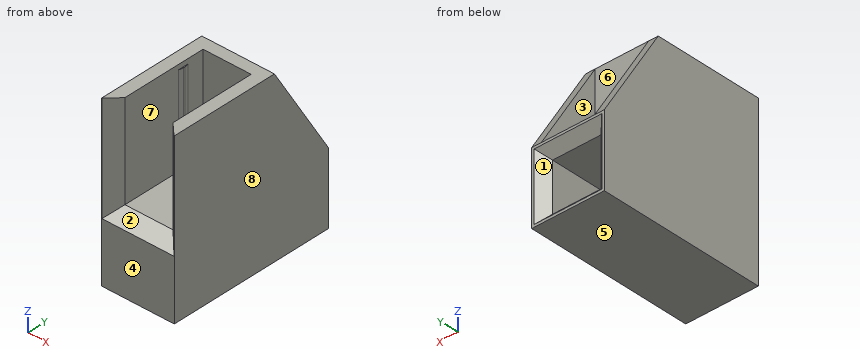
```python
from build123d import *

# Parameters (mm, degrees)
CROQUIS2_W               = 30.3
CROQUIS2_H               = 70
SALIENTE_EXTRUIR2_DEPTH  = 5
SALIENTE_EXTRUIR3_START  = -20
SALIENTE_EXTRUIR3_DEPTH  = 70
SALIENTE_EXTRUIR4_START  = -20
CROQUIS4_W               = 20.2
CROQUIS4_H               = 20.2
SALIENTE_EXTRUIR4_DEPTH  = 4
CHAFL_N4_SIZE            = 4
CROQUIS6_W               = 30.3
CROQUIS6_H               = 5
CROQUIS6_W_2             = 5.125
CROQUIS6_H_2             = 40.5
SALIENTE_EXTRUIR6_DEPTH  = 40
SALIENTE_EXTRUIR7_START  = -15.15
SALIENTE_EXTRUIR7_DEPTH  = 30.3
CROQUIS8_W               = 22.3
CROQUIS8_H               = 24.5
CORTAR_EXTRUIR1_DEPTH    = 40
CHAFL_N9_SIZE            = 5
SALIENTE_EXTRUIR9_DEPTH  = 0.4
REDONDEO3_R              = 5
SALIENTE_EXTRUIR10_DEPTH = 0.4
REDONDEO4_R              = 5


with BuildPart() as part:
    # Croquis2 → Saliente-Extruir2 (new body)
    with BuildSketch(Plane.XY):
        with Locations((0, 15)):
            Rectangle(CROQUIS2_W, CROQUIS2_H)
    extrude(amount=-SALIENTE_EXTRUIR2_DEPTH)

    # Croquis3 → Saliente-Extruir3 (add)
    with BuildSketch(Plane(origin=(0, 0, 0), x_dir=(1, 0, 0), z_dir=(0, 1, 0)).offset(SALIENTE_EXTRUIR3_START)):
        Polygon((-15.15, 30.25), (-15.15, 5), (-10.1, 5), (-10.1, 25.2), (10.1, 25.2), (10.1, 5), (15.15, 5), (15.15, 30.25), align=None)
    extrude(amount=SALIENTE_EXTRUIR3_DEPTH)

    # Croquis4 → Saliente-Extruir4 (add)
    with BuildSketch(Plane(origin=(0, 0, 0), x_dir=(1, 0, 0), z_dir=(0, 1, 0)).offset(SALIENTE_EXTRUIR4_START)):
        with Locations((0, 15.1)):
            Rectangle(CROQUIS4_W, CROQUIS4_H)
    extrude(amount=SALIENTE_EXTRUIR4_DEPTH)

    # Chaflán4
    chafl_n4_edges = [part.edges().sort_by_distance(p)[0] for p in [
        (0, 50, -5),
        (10.1, 50, -15.1),
        (0, 50, -25.2),
        (-10.1, 50, -15.1),
    ]]
    chamfer(chafl_n4_edges, length=CHAFL_N4_SIZE)

    # Croquis6 → Saliente-Extruir6 (add)
    with BuildSketch(Plane.XY):
        with Locations((0, 23)):
            Rectangle(CROQUIS6_W, CROQUIS6_H)
        with Locations((-12.5875, 0.25)):
            Rectangle(CROQUIS6_W_2, CROQUIS6_H_2)
        with Locations((12.5875, 0.25)):
            Rectangle(CROQUIS6_W_2, CROQUIS6_H_2)
    extrude(amount=SALIENTE_EXTRUIR6_DEPTH)

    # Croquis7 → Saliente-Extruir7 (add)
    with BuildSketch(Plane(origin=(0, 0, 0), x_dir=(0, 0, -1), z_dir=(1, 0, 0)).offset(SALIENTE_EXTRUIR7_START)):
        Polygon((-40, 25.5), (0, 50), (0, 25.5), align=None)
    extrude(amount=SALIENTE_EXTRUIR7_DEPTH)

    # Croquis8 → Cortar-Extruir1 (cut)
    with BuildSketch(Plane.XY):
        with Locations((0, 37.75)):
            Rectangle(CROQUIS8_W, CROQUIS8_H)
    extrude(amount=CORTAR_EXTRUIR1_DEPTH, mode=Mode.SUBTRACT)

    # Chaflán9
    chafl_n9_edges = [part.edges().sort_by_distance(p)[0] for p in [
        (0, -20, 0),
        (-10.025, -20, 20),
        (10.025, -20, 20),
    ]]
    chamfer(chafl_n9_edges, length=CHAFL_N9_SIZE)

    # Croquis22 → Saliente-Extruir9 (add)
    with BuildSketch(Plane(origin=(-10.025, 0, 0), x_dir=(0, 0, -1), z_dir=(1, 0, 0))):
        Polygon((-2, 13.75), (-10, 13.75), (-30, 13.75), (-38, 13.75), (-38, 9.25), (-30, 9.25), (-10, 9.25), (-2, 9.25), align=None)
    extrude(amount=SALIENTE_EXTRUIR9_DEPTH)

    # Redondeo3
    # the kernel refuses this fillet: 5 mm, written as the material it takes off along each edge
    with BuildSketch(Plane(origin=(-9.625, 9.25, 2), x_dir=(-1, 0, 0), z_dir=(0, 0, 1)), Plane(origin=(-9.625, 13.75, 42.898979486), x_dir=(-1, 0, 0), z_dir=(0, 0, -1))) as redondeo3_piece_1:
        with BuildLine():
            CenterArc((5, -1.959591794), REDONDEO3_R, 156.926081934, 23.073918066)
            Line((0, -1.959591794), (0, 0))
            Line((0, 0), (0.4, 0))
        make_face()
    extrude(amount=40.898979486, mode=Mode.SUBTRACT)

    # Croquis26 → Saliente-Extruir10 (add)
    with BuildSketch(Plane.ZY.offset(-10.025)):
        Polygon((10, 13.75), (2, 13.75), (2, 9.25), (10, 9.25), (30, 9.25), (38, 9.25), (38, 13.75), (30, 13.75), align=None)
    extrude(amount=SALIENTE_EXTRUIR10_DEPTH)

    # Redondeo4
    # the kernel refuses this fillet: 5 mm, written as the material it takes off along each edge
    with BuildSketch(Plane(origin=(9.625, 9.25, 42.898979486), x_dir=(1, 0, 0), z_dir=(0, 0, -1)), Plane(origin=(9.625, 13.75, 2), x_dir=(1, 0, 0), z_dir=(0, 0, 1))) as redondeo4_piece_1:
        with BuildLine():
            CenterArc((5, -1.959591794), REDONDEO4_R, 156.926081934, 23.073918066)
            Line((0, -1.959591794), (0, 0))
            Line((0, 0), (0.4, 0))
        make_face()
    extrude(amount=40.898979486, mode=Mode.SUBTRACT)


solid = part.part
```
Here's how the part is built. I have some questions about the finished solid (model axes, mm). Face numbers are marked on the shaded views. A direction names the side the tool comes from. Coordinates: 2 decimals unless noted, no trailing zeros. Write each loop counter-clockwise with the first axis right and the second up, starting at its lowest first coordinate (ties: lowest second). Pieces come first, ordered by that corner, then holes. Notation, with made-up numbers: (34.5, -7) -> (46.5, -7) arc R12 ccw to (46.5, 4) -> close; hole circle Ø5 at (31.5, -17). An arc over 180 degrees is marked (long way). Use a Markdown table: item, result. Add a question column.
(1) If we section it at C-C, the plane x = 8: Write out the boundary of the cut face in (y, z).
(2) If we section it at D-D, the plane z = 16: Write out the boundary of the cut face in (x, y) (3 decimals), and give its area (3 significant figures).
(3) I'm going to push flat-ended pins straight in: P1, Ø6, axis at x = -6.5, z = -15, coming from the +Y side; P2, Ø10, axis at x = -8, z = -21.5, coming from the +Y side; P3, Ø6, axis at x = 0, y = 14, coming from the +Z side. Where does each tip first touch, or does it pass through?
(4) We'd pull the mould along Y, two halves only. Please class the marked faces 6, 7 and 8: +Y half, -Y half, draft (parallel to the pull), parting line (faces both ways), or undercut.
(5) If we section it at A-A, the plane y = -12.5: Write out the boundary of the cut face in (x, z) (3 decimals), and give its area (3 significant figures).
(6) Please list where these lines run through material, in increasing order: line 1 (X direction, y = 42.5, z = 4.5); line 2 (Z direction, x = -6.5, y = 13); line 3 (X direction, y = 22.5, z = -8).
(7) For the marked faces 1, 2, 3, 4 and 5, which set-ups out of +Z, -Z, +X, -X, +Y, -Y let a thin tool reach every point of the face, with its end or its side?
(8) If we section it at B-B, the plane z = -24: Write out the boundary of the cut face in (x, y).
Outcome:
| question | item | result |
|---|---|---|
| 1 | outline | (-20, -30.25) -> (50, -30.25) -> (50, -29.2) -> (46, -25.2) -> (-16, -25.2) -> (-16, -5) -> (46, -5) -> (50, -1) -> (50, 0) -> (25.5, 0) -> (25.5, 40) -> (20.5, 40) -> (20.5, 0) -> (-15, 0) -> (-20, -5) -> close |
| 2 | outline | (-15.15, -20) -> (-15.025, -20) -> (-10.025, -15) -> (-10.025, 9.25) arc R5 ccw to (-9.625, 11.21) -> (-9.625, 11.79) arc R5 ccw to (-10.025, 13.75) -> (-10.025, 20.5) -> (10.025, 20.5) -> (10.025, 13.75) arc R5 ccw to (9.625, 11.79) -> (9.625, 11.21) arc R5 ccw to (10.025, 9.25) -> (10.025, -15) -> (15.025, -20) -> (15.15, -20) -> (15.15, 40.2) -> (11.15, 40.2) -> (11.15, 25.5) -> (-11.15, 25.5) -> (-11.15, 40.2) -> (-15.15, 40.2) -> close |
| 2 | area | 662 mm^2 |
| 3 | P1 | stops at y = -16 |
| 3 | P2 | stops at y = 48.9 |
| 3 | P3 | stops at z = 0 |
| 4 | face 6 | +Y half |
| 4 | face 7 | undercut |
| 4 | face 8 | draft |
| 5 | outline | (-15.15, -30.25) -> (15.15, -30.25) -> (15.15, 40) -> (10.025, 40) -> (10.025, 0) -> (-10.025, 0) -> (-10.025, 40) -> (-15.15, 40) -> close; hole (-10.1, -25.2) -> (10.1, -25.2) -> (10.1, -5) -> (-10.1, -5) -> close |
| 5 | area | 919 mm^2 |
| 6 | line 1 | x = -15.15 to -11.15, 11.15 to 15.15 |
| 6 | line 2 | z = -30.25 to -25.2, -5 to 0 |
| 6 | line 3 | x = -15.15 to -10.1, 10.1 to 15.15 |
| 7 | face 1 | +Y |
| 7 | face 2 | +Z, -Y |
| 7 | face 3 | +Z, +Y |
| 7 | face 4 | +Z, -Z, +X, -X, -Y |
| 7 | face 5 | -Z, +X, -X, +Y, -Y |
| 8 | outline | (-15.15, -20) -> (15.15, -20) -> (15.15, 50) -> (14.1, 50) -> (10.1, 46) -> (10.1, -16) -> (-10.1, -16) -> (-10.1, 46) -> (-14.1, 50) -> (-15.15, 50) -> close |
